Geometry check sheet. Reference: the model listing, model coordinates, mm. Face numbers are marked on the shaded views. A direction names the side the tool comes from. Coordinates: 2 decimals unless noted, no trailing zeros. Loops run counter-clockwise (first coordinate to the right, second up) from the corner with the lowest first, then second, coordinate; pieces in that order, holes last.
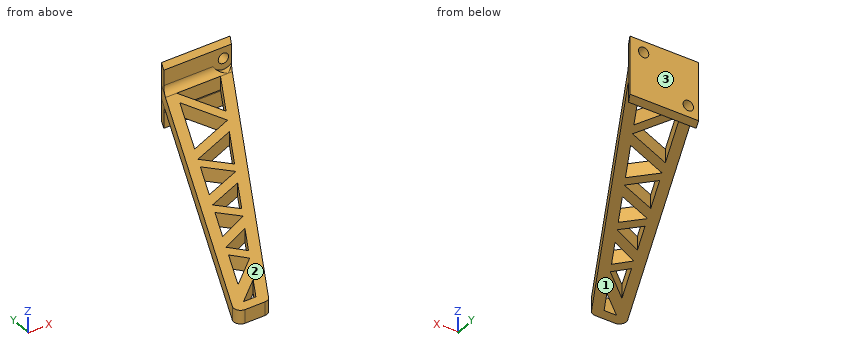
from build123d import *

# Parameters (mm, degrees)
BOSS_EXTRUDE1_DEPTH             = 4
SKETCH2_W                       = 20
SKETCH2_H                       = 17
BOSS_EXTRUDE2_DEPTH             = 3
CUT_EXTRUDE1_DEPTH              = 104.490337713
CUT_EXTRUDE1_DEPTH_BACK         = 104.490337713
BOSS_EXTRUDE3_REACH             = 105.49
BOSS_EXTRUDE3_DIRECTION_2_REACH = 105.49
FILLET2_START                   = -12.222222222
FILLET2_DEPTH                   = 20.555555555
FILLET2_START_2                 = -6.5
FILLET2_2_DEPTH                 = 17
CUT_EXTRUDE2_DEPTH              = 104.490337713
CUT_EXTRUDE2_DEPTH_BACK         = 104.490337713
SKETCH4_R                       = 1.5
FILLET1_R                       = 2
SKETCH8_R                       = 3.25
CUT_EXTRUDE5_DEPTH              = 2


with BuildPart() as part:
    # Sketch1 → Boss-Extrude1 (new body)
    with BuildSketch(Plane.XY):
        Polygon((-10, 0), (10, 0), (-40, -90), (-50, -90), align=None)
        Polygon((-8.939269622, -5), (3.790345509, -5), (-3.431876714, -18), align=None, mode=Mode.SUBTRACT)
        Polygon((-10.607355622, -8.753193502), (-18.717047399, -27), (-5.280384607, -21.327314208), align=None, mode=Mode.SUBTRACT)
        Polygon((-7.643825511, -25.581507835), (-14.336143532, -37.627680274), (-20.498621264, -31.008541196), align=None, mode=Mode.SUBTRACT)
        Polygon((-21.823082205, -33.988578312), (-26.698028096, -44.957206566), (-15.867976064, -40.384978831), align=None, mode=Mode.SUBTRACT)
        Polygon((-18.231416968, -44.639172459), (-23.566710848, -54.242701442), (-28.47960196, -48.965747762), align=None, mode=Mode.SUBTRACT)
        Polygon((-29.804062901, -51.945784878), (-33.981685193, -61.345435036), (-25.09854338, -57), align=None, mode=Mode.SUBTRACT)
        Polygon((-45.383714066, -87), (-41.765210047, -87), (-38.207091023, -80.595385758), align=None, mode=Mode.SUBTRACT)
        Polygon((-27.646340017, -61.586033947), (-32.225825485, -69.829107788), (-35.878360761, -65.612955064), align=None, mode=Mode.SUBTRACT)
        Polygon((-37.22421022, -68.641116347), (-42.421865314, -80.335840308), (-33.776674606, -72.620636206), align=None, mode=Mode.SUBTRACT)
    extrude(amount=BOSS_EXTRUDE1_DEPTH)

    # Sketch2 → Boss-Extrude2 (add)
    with BuildSketch(Plane(origin=(0, 0, 0), x_dir=(1, 0, 0), z_dir=(0, 1, 0))):
        with Locations((0, -2)):
            Rectangle(SKETCH2_W, SKETCH2_H)
    extrude(amount=-BOSS_EXTRUDE2_DEPTH)

    # Sketch3 → Cut-Extrude1 (cut, two sides: drawn at the far end of the back side and taken through both)
    with BuildSketch(Plane.XY.offset(4).offset(-CUT_EXTRUDE1_DEPTH_BACK)):
        Polygon((8.333333333, -3), (10, 0), (10, -3), align=None)
    extrude(amount=CUT_EXTRUDE1_DEPTH + CUT_EXTRUDE1_DEPTH_BACK, mode=Mode.SUBTRACT)

    # Boss-Extrude3: up to this face of the body (flat: up to its plane)
    boss_extrude3_end = Plane(part.part.faces().sort_by_distance((-0.410628019, -1.47826087, 10.5))[0])
    # Sketch7 → Boss-Extrude3 (add, up to the picked face)
    with BuildSketch(Plane.XY.offset(4), mode=Mode.PRIVATE) as boss_extrude3_sk1:
        Polygon((-10, -3), (-11.333333333, -3), (-10, 0), align=None)
    boss_extrude3_tool1 = split(extrude(boss_extrude3_sk1.sketch, amount=BOSS_EXTRUDE3_REACH, mode=Mode.PRIVATE), bisect_by=boss_extrude3_end, keep=Keep.BOTH, mode=Mode.PRIVATE)
    add(boss_extrude3_tool1.solids().sort_by(Axis((-10.444444, -2, 4), (0, 0, 1)))[0])

    # Boss-Extrude3 direction 2: up to this face of the body (flat: up to its plane)
    boss_extrude3_direction_2_end = Plane(part.part.faces().sort_by_distance((-0.410628019, -1.47826087, -6.5))[0])
    # Sketch7 → Boss-Extrude3 direction 2 (add, up to the picked face)
    with BuildSketch(Plane.XY.offset(4), mode=Mode.PRIVATE) as boss_extrude3_direction_2_sk1:
        Polygon((-10, -3), (-11.333333333, -3), (-10, 0), align=None)
    boss_extrude3_direction_2_tool1 = split(extrude(boss_extrude3_direction_2_sk1.sketch, amount=-BOSS_EXTRUDE3_DIRECTION_2_REACH, mode=Mode.PRIVATE), bisect_by=boss_extrude3_direction_2_end, keep=Keep.BOTH, mode=Mode.PRIVATE)
    add(boss_extrude3_direction_2_tool1.solids().sort_by(Axis((-10.444444, -2, 4), (0, 0, -1)))[0])

    # Fillet2: read off the stored shape, not the designer's step
    # Fillet2 outline → Fillet2 (add)
    with BuildSketch(Plane.YZ.offset(FILLET2_START)):
        with BuildLine():
            Line((-3, 4), (-3, 6))
            ThreePointArc((-3, 6), (-3.585786438, 4.585786438), (-5, 4))
            Line((-5, 4), (-3, 4))
        make_face()
        with BuildLine():
            ThreePointArc((-5, 0), (-3.585786438, -0.585786438), (-3, -2))
            Line((-3, -2), (-3, 0))
            Line((-3, 0), (-5, 0))
        make_face()
    extrude(amount=FILLET2_DEPTH)

    # Fillet2 2 outline → Fillet2 2 (cut)
    with BuildSketch(Plane.XY.offset(FILLET2_START_2)):
        Polygon((10, -1), (9.444444444, -1), (8.333333333, -3), (6.666666667, -6), (10, -6), align=None)
        Polygon((-12.222222222, -5), (-11.333333333, -3), (-12.222222222, -3), align=None)
    extrude(amount=FILLET2_2_DEPTH, mode=Mode.SUBTRACT)

    # Sketch4 → Cut-Extrude2 (cut, two sides: drawn at the far end of the back side and taken through both)
    with BuildSketch(Plane(origin=(0, 0, 0), x_dir=(1, 0, 0), z_dir=(0, 1, 0)).offset(-CUT_EXTRUDE2_DEPTH_BACK)):
        with Locations(Location((-7, 3.25, 0), (0, 0, 236.442690238))):
            Circle(SKETCH4_R)
        with Locations(Location((6, -7.25, 0), (0, 0, 123.557309765))):
            Circle(SKETCH4_R)
    extrude(amount=CUT_EXTRUDE2_DEPTH + CUT_EXTRUDE2_DEPTH_BACK, mode=Mode.SUBTRACT)

    # Fillet1
    fillet1_edges = [part.edges().sort_by_distance(p)[0] for p in [
        (-40, -90, 2),
        (-50, -90, 2),
    ]]
    fillet(fillet1_edges, radius=FILLET1_R)

    # Sketch8 → Cut-Extrude5 (cut)
    with BuildSketch(Plane.XZ.offset(3)):
        with Locations((-7, -3.25)):
            Circle(SKETCH8_R)
        with Locations((6, 7.25)):
            Circle(SKETCH8_R)
    extrude(amount=CUT_EXTRUDE5_DEPTH, mode=Mode.SUBTRACT)


solid = part.part
1) Section check A-A on z = 7.25. Record the cut outline in (x, y), and give its area (3 significant figures).
Data:
outline: (-11.33, -3) - (4.5, -3) - (4.5, 0) - (-10, 0) - close; (7.5, -3) - (8.33, -3) - (10, 0) - (7.5, 0) - close
area: 50.5 mm2
2) Section check B-B on y = -53. Record the cut outline in (x, z), and give its area (3 significant figures).
Data:
outline: (-33.56, 0) - (-30.27, 0) - (-30.27, 4) - (-33.56, 4) - close; (-28.82, 0) - (-24.72, 0) - (-24.72, 4) - (-28.82, 4) - close; (-22.88, 0) - (-19.44, 0) - (-19.44, 4) - (-22.88, 4) - close
area: 43.3 mm2
3) Material ranges on probe 1 along Z at (x, y) = (6, -2.15); probe 2 along Z at (x, y) = (-11.5, -7); probe 3 along Y at (x, z) = (-16.5, 3) (3 decimals), recorded low to high.
Data:
probe 1: z = -6.5 to 5.75, 8.75 to 10.5
probe 2: z = 0 to 4
probe 3: y = -47.7 to -40.652, -39.706 to -35.303, -29.32 to -26.064, -22.012 to -14.625
4) Access from +Z, -Z, +X, -X, +Y, -Y to the whole of each face (thin tool, end or side, straight path). Record for the marked faces 1, 2 and 3.
Data:
face 1: -Z, +X, -X, -Y
face 2: +Z, +X, -X, -Y
face 3: +Z, -Z, +X, -X, +Y
5) Section check C-C on x = 0.5. Record the cut outline in (y, z), and give its area (3 significant figures).
Data:
outline: (-17.1, 0) - (-10.92, 0) - (-10.92, 4) - (-17.1, 4) - close; (-5, 0) arc R2 cw to (-3, -2) - (-3, -6.5) - (0, -6.5) - (0, 10.5) - (-3, 10.5) - (-3, 6) arc R2 cw to (-5, 4) - close
area: 85.4 mm2
6) Depth check by flat-ended pin: pin 1 (4 mm diameter, centred on y = -60, z = 1.5, fed in from +X); pin 2 (5 mm diameter, centred on x = 6, z = 7.25, fed in from -Y); pin 3 (5 mm diameter, centred on x = -7, z = -3.25, fed in from +Y); pin 4 (1.8 mm diameter, centred on x = -44.5, z = 3, fed in from +Y). Enter the tip coordinate at first touch or a pass-through.
Data:
pin 1: stops at x = -22.22
pin 2: stops at y = -3
pin 3: stops at y = 0
pin 4: stops at y = -75.6
